```python
from build123d import *

# Parameters (mm, degrees)
SKETCH1_R           = 1.75
BOSS_EXTRUDE1_DEPTH = 25
FILLET2_R           = 3
FILLET3_R           = 3
SKETCH2_R           = 1
CUT_EXTRUDE1_DEPTH  = 10


with BuildPart() as part:
    # Sketch1 → Boss-Extrude1 (new body)
    with BuildSketch(Plane(origin=(0, 0, 0), x_dir=(1, 0, 0), z_dir=(0, 1, 0))):
        with BuildLine():
            Line((49.859310292, 3.748223209), (43.664405044, 3.223270017))
            ThreePointArc((43.664405044, 3.223270017), (40.162533858, -17.433892609), (27.463538801, -34.098735665))
            Line((27.463538801, -34.098735665), (-27.821692195, -34.098735665))
            ThreePointArc((-27.821692195, -34.098735665), (-40.425237601, -17.394553614), (-43.88915269, 3.242315021))
            Line((-43.88915269, 3.242315021), (-49.859310292, 3.748223209))
            ThreePointArc((-49.859310292, 3.748223209), (-44.960475989, -21.875913669), (-27.821692195, -41.544595839))
            Line((-27.821692195, -41.544595839), (27.463538801, -41.782221537))
            ThreePointArc((27.463538801, -41.782221537), (44.866035011, -22.06895789), (49.859310292, 3.748223209))
        make_face()
        with Locations(Location((-47, 0, 0), (0, 0, 270))):
            Circle(SKETCH1_R, mode=Mode.SUBTRACT)
        with Locations(Location((47, 0, 0), (0, 0, 90))):
            Circle(SKETCH1_R, mode=Mode.SUBTRACT)
    extrude(amount=BOSS_EXTRUDE1_DEPTH)

    # Fillet2
    fillet2_edges = [part.edges().sort_by_distance(p)[0] for p in [
        (43.664405044, 12.5, -3.223270017),
        (49.859310292, 12.5, -3.748223209),
        (-43.88915269, 12.5, -3.242315021),
    ]]
    fillet(fillet2_edges, radius=FILLET2_R)

    # Fillet3
    # the kernel refuses this fillet: 3 mm, written as the material it takes off along each edge
    with BuildSketch(Plane(origin=(-49.859310292, -8.061567981, -3.748223209), x_dir=(-0.04276994163543241, 0, 0.9990849473856073), z_dir=(0, 1, 0))) as fillet3_piece_1:
        with BuildLine():
            CenterArc((3.127888377, 2.998439861), FILLET3_R, 177.607640596, 94.240255032)
            Line((0.13050316, 3.123667112), (0, 0))
            ThreePointArc((0, 0), (1.612313596, -0.026002313), (3.224627192, 0))
        make_face()
    extrude(amount=41.123135962, mode=Mode.SUBTRACT)

    # Sketch2 → Cut-Extrude1 (cut)
    with BuildSketch(Plane(origin=(-0.179076697, 0, 41.663408688), x_dir=(0.9999907629660516, 0, 0.004298137105095237), z_dir=(-0.004298137105095237, 0, 0.9999907629660516))):
        with Locations((10, 2.5)):
            Circle(SKETCH2_R)
        with Locations((-10, 2.5)):
            Circle(SKETCH2_R)
        with Locations((10, 22.5)):
            Circle(SKETCH2_R)
        with Locations((-10, 22.5)):
            Circle(SKETCH2_R)
    extrude(amount=-CUT_EXTRUDE1_DEPTH, mode=Mode.SUBTRACT)


solid = part.part
```
Part model, mm, in its own coordinate system. Round coordinates to 2 decimals unless told otherwise and drop trailing zeros. Write each loop counter-clockwise with the first axis right and the second up, starting at its lowest first coordinate (ties: lowest second). Pieces come first, ordered by that corner, then holes. Notation, with made-up numbers: M -26,38.5 L 32,38.5 A25 cw 32,77.5 Z; hole C 38,58.5 d11. An arc over 180 degrees is marked long. One line per question, with ' | ' between items.
(1) Saw through at D-D on x = -38. Write the cut outline in (y, z), then the cut area to 3 significant figures.
Answer key:
outline: M 0,22.2 L 25,22.2 L 25,32.5 L 0,32.5 Z | area: 257 mm^2
(2) Saw through at A-A on z = 18.5. Write the cut outline in (x, y), then the cut area to 3 significant figures.
Answer key:
outline: M -46.45,0 L -39.93,0 L -39.93,25 L -46.45,25 Z; M 39.68,0 L 46.45,0 L 46.45,25 L 39.68,25 Z | area: 332 mm^2
(3) Probe line 1 along X through (y, z) = (12, 0); line 2 along Z through (x, y) = (7, 24.25); line 3 along Z through (x, y) = (25.5, 4.25). List the from-to ranges inside material, lowest first.
Answer key:
line 1: x = -50 to -48.75, -45.25 to -44.01, 43.78 to 45.25, 48.75 to 50 | line 2: z = 34.1 to 41.69 | line 3: z = 34.1 to 41.77
(4) Pin check, flat tips, straight feed: pin 1 (10 mm diameter, centred on x = -14, y = 18.5, fed in from -Z); pin 2 (4 mm diameter, centred on x = -28, y = 17, fed in from +Z); pin 3 (10 mm diameter, centred on y = 10.5, z = 23.5, fed in from +X); pin 4 (8 mm diameter, centred on x = -32.5, z = 28, fed in from +Y). Stop position of each tip, or through.
Answer key:
pin 1: stops at z = 34.1 | pin 2: stops at z = 41.55 | pin 3: stops at x = 46.45 | pin 4: stops at y = 25
(5) Saw through at B-B on z = 0.5. Write the cut outline in (x, y), then the cut area to 3 significant figures.
Answer key:
outline: M -50,0 L -48.68,0 L -48.68,25 L -50,25 Z; M -45.32,0 L -44.01,0 L -44.01,25 L -45.32,25 Z; M 43.78,0 L 45.32,0 L 45.32,25 L 43.78,25 Z; M 48.68,0 L 50,0 L 50,25 L 48.68,25 Z | area: 138 mm^2
(6) Two-plate mould, pull along X, no slides. Class faces 1 (the face through (-48.71, 12.32, -0.38)), 2 (the face through (43.965, 12.325, 23.813)), 3 (the face through (0, 25, 36)): released by +X, released by -X, zero draft, split by the parting line, or undercut.
Answer key:
face 1: undercut | face 2: released by +X | face 3: zero draft
(7) Saw through at C-C on y = 7. Write the cut outline in (x, z), then the cut area to 3 significant figures.
Answer key:
outline: M -50,-0.53 A3 ccw -46.75,-3.48 A3 ccw -44.01,-0.46 A44.01 cw -27.82,34.1 L 27.46,34.1 A43.78 cw 43.78,-0.45 A3 ccw 46.53,-3.47 L 46.74,-3.48 A3 ccw 50,-0.53 A50 ccw 27.46,41.78 L -27.82,41.54 A50 ccw Z; hole C -47,0 d3.5; hole C 47,0 d3.5 | area: 973 mm^2
